Check sheet for the modelled part. Datum: model origin and axes. Units: mm. A direction names the side the tool comes from. Give positions to 0.01 mm unless a question says otherwise; leave off trailing zeros. Order: outer loops, then holes, each group sorted by start corner. A loop starts at its lowest first (then second) coordinate and runs counter-clockwise, first axis right, second up.
Solid Edge part; units mm, degrees
sketch "Sketch1" plane through (0, 0, 0) normal (0, -1, 0) x (1, 0, 0)
  line L0 (-53.3125, 21.0114) -> (66.6875, 21.0114)
  line L1 (66.6875, 21.0114) -> (66.6875, -28.9886)
  line L2 (66.6875, -28.9886) -> (-53.3125, -28.9886)
  line L3 (-53.3125, -28.9886) -> (-53.3125, 21.0114)
extrude "Protrusion1" add sketch "Sketch1" against normal blind 140
hole "Hole1" at (36.6875, 0, -3.9886) direction (0, 1, 0) diameter 20 end up to next
hole "Hole_2" at (-23.3125, 0, -3.9886) direction (0, 1, 0) diameter 20 end up to next
hole "Hole_3" at (6.6875, 70, 21.0114) direction (0, 0, -1) diameter 20 end up to next counterbore diameter 36 counterbore depth 12
properties part number "C-3701" material "Steel"
Q1. Go/stop test with a flat-tipped pin: P1, Ø18, axis at x = -23.31, z = -3.99, coming from the -Y side. Record where the tip stops, or that it passes through.
Q2. Sectioned sample at C-C, the plane x = 41.5. Record the cut outline in (y, z), plus the area to 3 significant figures.
Q3. Tool access check on faces 5 (the flat face through (14, 62, 9.011)), 6 (the flat face through (8, 140, -4)). Record the directions out of +Z, -Z, +X, -X, +Y, -Y that give a thin tool (end or side, any length) a straight path to the whole face; none if there is none.
Q4. Draft check along X on faces 1 (the flat face through (-53.312, 69, -4)), 2 (the cylindrical face through (5.896, 87.983, 14.927)), 3 (the cylindrical face through (7.13, 79.99, -9.72)), 4 (the flat face through (21, 69, -28.989)). Enter one of: pulls with the +X half, pulls with the -X half, needs draft (parallel to the pull), parting line crosses it, or undercut.
Q5. Sectioned sample at B-B, the plane y = 70. Record the cut outline in (x, z).
Q6. Sectioned sample at D-D, the plane y = 85. Record the cut outline in (x, z), plus the area to 3 significant figures.
Q7. Sectioned sample at A-A, the plane z = -0.5. Record the cut outline in (x, y), plus the area to 3 significant figures.
Q8. Material ranges on line 1 (X direction, y = 70, z = 15); line 2 (X direction, y = 122, z = -6); line 3 (Z direction, x = 36.5, y = 37.5), recorded low to high.
Filled in:
1. P1: passes through
2. outline: (0, -28.99) - (140, -28.99) - (140, -12.75) - (0, -12.75) - close; (0, 4.78) - (140, 4.78) - (140, 21.01) - (0, 21.01) - close
2. area: 4,550 mm2
3. face 5: +Z
3. face 6: +Z, -Z, +X, -X, +Y
4. face 1: pulls with the -X half
4. face 2: undercut
4. face 3: undercut
4. face 4: needs draft
5. outline: (-53.31, -28.99) - (-3.31, -28.99) - (-3.31, 9.01) - (-11.31, 9.01) - (-11.31, 21.01) - (-53.31, 21.01) - close; (16.69, -28.99) - (66.69, -28.99) - (66.69, 21.01) - (24.69, 21.01) - (24.69, 9.01) - (16.69, 9.01) - close; hole circle Ø20 at (-23.31, -3.99); hole circle Ø20 at (36.69, -3.99)
6. outline: (-53.31, -28.99) - (66.69, -28.99) - (66.69, 21.01) - (16.64, 21.01) - (16.64, 9.01) - (-3.26, 9.01) - (-3.26, 21.01) - (-53.31, 21.01) - close; hole circle Ø20 at (-23.31, -3.99); hole circle Ø20 at (36.69, -3.99)
6. area: 5,130 mm2
7. outline: (-53.31, 0) - (-32.68, 0) - (-32.68, 140) - (-53.31, 140) - close; (-13.94, 0) - (27.32, 0) - (27.32, 140) - (-13.94, 140) - close; (46.06, 0) - (66.69, 0) - (66.69, 140) - (46.06, 140) - close; hole circle Ø20 at (6.69, 70)
7. area: 11,200 mm2
8. line 1: x = -53.31 to -11.31, 24.69 to 66.69
8. line 2: x = -53.31 to -33.11, -13.52 to 26.89, 46.48 to 66.69
8. line 3: z = -28.99 to -13.99, 6.01 to 21.01
